The listing builds one solid part. Answer for the finished solid, in the listing's coordinates (mm). Face numbers are marked on the shaded views. A direction names the side the tool comes from. Round coordinates to 2 decimals unless told otherwise and drop trailing zeros. Order: outer loops, then holes, each group sorted by start corner. A loop starts at its lowest first (then second) coordinate and runs counter-clockwise, first axis right, second up. Notation, with made-up numbers: (-1.75, 19) - (11.25, 19) arc R26 cw to (11.25, 51) - close; hole circle Ø9 at (83.25, 75.25). An arc over 180 degrees is marked (long way). One line per item, written item: value. Start each with the question number.
1. Section A-A, the plane y = 23.5 is taken. Give the vertices of the cut face in (x, z).
2. A tool of negligible diameter and unlimited length cuts with its end or side. For the marked faces 1, 2 and 3, from which of +Z, -Z, +X, -X, +Y, -Y can it reach the whole face along a straight path? Write none if from no direction.
3. Section C-C, the plane y = 7 is taken. Give the vertices of the cut face in (x, z), then the cut area to 3 significant figures.
4. Flat-ended cylindrical pins translate along their axes: P1, Ø5, axis at y = 66, z = -5, coming from the +X side; P2, Ø2.5, axis at x = 1, y = 19.5, coming from the +Z side; P3, Ø12, axis at y = 31, z = -3.5, coming from the -X side. Find the tip coordinate at first contact, or state that the pin passes through.
5. Straight lines are drawn through the part: line 1 (Y direction, x = -4.75, z = -6.75); line 2 (Y direction, x = 1.5, z = 6.75); line 3 (X direction, y = 51.5, z = -1.5). For each, find the intervals that lie inside material, in ascending order.
6. Section B-B, the plane z = 8.25 is taken. Give the vertices of the cut face in (x, y).
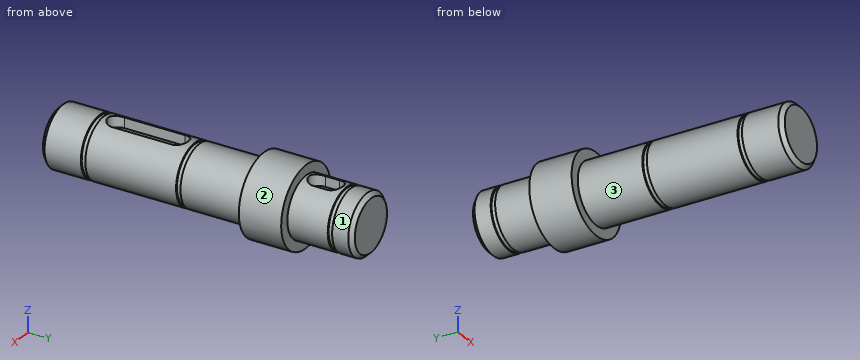
from build123d import *

# Parameters (mm, degrees)
SFAZOWANIE1_SIZE           = 1
WYTNIJ_WYCI_GNI_CIE1_DEPTH = 3


with BuildPart() as part:
    # Szkic1 → Obrót1 (revolve)
    with BuildSketch(Plane.XY, mode=Mode.PRIVATE) as obr_t1_sk:
        Polygon((0, 0), (-7.5, 0), (-7.5, 10), (-7.15, 10), (-7.15, 11.1), (-7.5, 11.1), (-7.5, 33.6), (-7.15, 33.6), (-7.15, 34.7), (-7.5, 34.7), (-7.5, 50.7), (-10, 50.7), (-10, 61.2), (-7.5, 61.2), (-7.5, 71.2), (-7.15, 71.2), (-7.15, 72.3), (-7.5, 72.3), (-7.5, 77.3), (0, 77.3), align=None)
    revolve(obr_t1_sk.sketch.rotate(Axis((0, 0, 0), (0, 1, 0)), 270), axis=Axis((0, 0, 0), (0, 1, 0)))

    # Sfazowanie1
    sfazowanie1_edges = [part.edges().sort_by_distance(p)[0] for p in [
        (0, 77.3, 7.5),
        (0, 0, 7.5),
    ]]
    chamfer(sfazowanie1_edges, length=SFAZOWANIE1_SIZE)

    # Szkic2 → Wytnij-wyciągnięcie1 (cut)
    with BuildSketch(Plane.XY.offset(7.5)):
        with BuildLine():
            Line((-2.5, 14.637705083), (-2.5, 29.637705083))
            ThreePointArc((-2.5, 29.637705083), (0, 32.137705083), (2.5, 29.637705083))
            Line((2.5, 29.637705083), (2.5, 14.637705083))
            ThreePointArc((2.5, 14.637705083), (0, 12.137705083), (-2.5, 14.637705083))
        make_face()
        with BuildLine():
            Line((-2.5, 64.45), (-2.5, 67.95))
            ThreePointArc((-2.5, 67.95), (0, 70.45), (2.5, 67.95))
            Line((2.5, 67.95), (2.5, 64.45))
            ThreePointArc((2.5, 64.45), (0, 61.95), (-2.5, 64.45))
        make_face()
    extrude(amount=-WYTNIJ_WYCI_GNI_CIE1_DEPTH, mode=Mode.SUBTRACT)


solid = part.part
Answer list:
1. outline: (-2.5, 4.5) - (-2.5, 7.07) arc R7.5 ccw (long way) to (2.5, 7.07) - (2.5, 4.5) - close
2. face 1: +Y
2. face 2: +Y, -Y
2. face 3: -Y
3. outline: circle Ø15 at (0, 0)
3. area: 177 mm²
4. P1: stops at x = 7.07
4. P2: stops at z = 4.5
4. P3: stops at x = -7.5
5. line 1: y = 50.7 to 61.2
5. line 2: y = 0.41 to 12.64, 31.64 to 62.45, 69.95 to 76.89
5. line 3: x = -9.89 to 9.89
6. outline: (-5.65, 50.7) - (5.65, 50.7) - (5.65, 61.2) - (-5.65, 61.2) - close
